from build123d import *

# Parameters (mm, degrees)
SKETCH1_W           = 250
SKETCH1_H           = 200
BOSS_EXTRUDE1_DEPTH = 3
SKETCH3_R           = 2
CUT_EXTRUDE2_DEPTH  = 3
CUT_EXTRUDE3_DEPTH  = 10


with BuildPart() as part:
    # Sketch1 → Boss-Extrude1 (new body)
    with BuildSketch(Plane.XY):
        Rectangle(SKETCH1_W, SKETCH1_H)
    extrude(amount=BOSS_EXTRUDE1_DEPTH)

    # Sketch3 → Cut-Extrude2 (cut)
    with BuildSketch(Plane.XY.offset(3)):
        with Locations((-85, 85)):
            Circle(SKETCH3_R)
        with Locations((-85, -85)):
            Circle(SKETCH3_R)
        with Locations((-85, -425)):
            Circle(SKETCH3_R)
        with Locations((85, -425)):
            Circle(SKETCH3_R)
        with Locations(Location((85, -85, 0), (0, 0, 180))):
            Circle(SKETCH3_R)
        with Locations(Location((85, 85, 0), (0, 0, 180))):
            Circle(SKETCH3_R)
    extrude(amount=-CUT_EXTRUDE2_DEPTH, mode=Mode.SUBTRACT)

    # Sketch4 → Cut-Extrude3 (cut)
    with BuildSketch(Plane(origin=(0, 0, 0), x_dir=(-1, 0, 0), z_dir=(0, 0, -1))):
        with BuildLine():
            Line((-99, -17), (-71, -17))
            ThreePointArc((-71, -17), (-69.585786438, -17.585786438), (-69, -19))
            Line((-69, -19), (-69, -53))
            ThreePointArc((-69, -53), (-69.585786438, -54.414213562), (-71, -55))
            Line((-71, -55), (-99, -55))
            ThreePointArc((-99, -55), (-100.414213562, -54.414213562), (-101, -53))
            Line((-101, -53), (-101, -19))
            ThreePointArc((-101, -19), (-100.414213562, -17.585786438), (-99, -17))
        make_face()
        with BuildLine():
            Line((69, -19), (69, -53))
            ThreePointArc((69, -53), (69.585786438, -54.414213562), (71, -55))
            Line((71, -55), (99, -55))
            ThreePointArc((99, -55), (100.414213562, -54.414213562), (101, -53))
            Line((101, -53), (101, -19))
            ThreePointArc((101, -19), (100.414213562, -17.585786438), (99, -17))
            Line((99, -17), (71, -17))
            ThreePointArc((71, -17), (69.585786438, -17.585786438), (69, -19))
        make_face()
    extrude(amount=-CUT_EXTRUDE3_DEPTH, mode=Mode.SUBTRACT)


solid = part.part
Here's how the part is built. I have some questions about the finished solid (model axes, mm). Round coordinates to 2 decimals unless told otherwise and drop trailing zeros. Order: outer loops, then holes, each group sorted by start corner. A loop starts at its lowest first (then second) coordinate and runs counter-clockwise, first axis right, second up. Notation, with made-up numbers: (81, 48) -> (123, 48) arc R10 ccw to (123, 60) -> close; hole circle Ø5 at (45, -25). An arc over 180 degrees is marked (long way). Return JSON: item names as keys, results as strings.
Q1. If we section it at C-C on x = 76: List the corners of the cut face in (y, z) for me.
Filled sheet:
{"outline": "(-100, 0) -> (-55, 0) -> (-55, 3) -> (-100, 3) -> close; (-17, 0) -> (100, 0) -> (100, 3) -> (-17, 3) -> close"}
Q2. I need wall thicknesses on line 1 along Y through (x, z) = (-85, 0.95); line 2 along X through (y, z) = (-30.5, 2.2); line 3 along Y through (x, z) = (96.5, 0.8). Which ranges of each line are inside material? Lowest first, please. Write a range as from..to.
Filled sheet:
{"line 1": "y = -100..-87, -83..-55, -17..83, 87..100", "line 2": "x = -125..-101, -69..69, 101..125", "line 3": "y = -100..-55, -17..100"}
Q3. If we section it at A-A on y = -37: List the corners of the cut face in (x, z) for me, plus the area to 3 significant figures.
Filled sheet:
{"outline": "(-125, 0) -> (-101, 0) -> (-101, 3) -> (-125, 3) -> close; (-69, 0) -> (69, 0) -> (69, 3) -> (-69, 3) -> close; (101, 0) -> (125, 0) -> (125, 3) -> (101, 3) -> close", "area": "558 mm^2"}
Q4. If we section it at B-B on z = 0.5: List the corners of the cut face in (x, y) for me, plus the area to 3 significant figures.
Filled sheet:
{"outline": "(-125, -100) -> (125, -100) -> (125, 100) -> (-125, 100) -> close; hole (-101, -53) arc R2 ccw to (-99, -55) -> (-71, -55) arc R2 ccw to (-69, -53) -> (-69, -19) arc R2 ccw to (-71, -17) -> (-99, -17) arc R2 ccw to (-101, -19) -> close; hole circle Ø4 at (-85, -85); hole circle Ø4 at (-85, 85); hole (69, -53) arc R2 ccw to (71, -55) -> (99, -55) arc R2 ccw to (101, -53) -> (101, -19) arc R2 ccw to (99, -17) -> (71, -17) arc R2 ccw to (69, -19) -> close; hole circle Ø4 at (85, -85); hole circle Ø4 at (85, 85)", "area": "47,500 mm^2"}
Q5. For pin 1 Ø3 at (x, y) = (85, -85) entering from +Z, with a flat end and sliding along its axis, tell me the tip position at first contact or that it passes through.
Filled sheet:
{"pin 1": "passes through"}
